```python
from build123d import *

# Parameters (mm, degrees)
SKETCH1_R           = 35
BOSS_EXTRUDE1_DEPTH = 170
SKETCH4_R           = 35
BOSS_EXTRUDE2_DEPTH = 85
SKETCH5_R           = 32.5
CUT_EXTRUDE2_DEPTH  = 85
SKETCH2_R           = 32.5
CUT_EXTRUDE3_DEPTH  = 194.261480901


with BuildPart() as part:
    # Sketch1 → Boss-Extrude1 (new body)
    with BuildSketch(Plane(origin=(0, 0, 0), x_dir=(0, 0, -1), z_dir=(1, 0, 0))):
        Circle(SKETCH1_R)
    extrude(amount=-BOSS_EXTRUDE1_DEPTH)

    # Sketch4 → Boss-Extrude2 (add)
    with BuildSketch(Plane.XY):
        with Locations((-85, 0)):
            Circle(SKETCH4_R)
    extrude(amount=-BOSS_EXTRUDE2_DEPTH)

    # Sketch5 → Cut-Extrude2 (cut)
    with BuildSketch(Plane(origin=(0, 0, -85), x_dir=(-1, 0, 0), z_dir=(0, 0, -1))):
        with Locations((85, 0)):
            Circle(SKETCH5_R)
    extrude(amount=-CUT_EXTRUDE2_DEPTH, mode=Mode.SUBTRACT)

    # Sketch2 → Cut-Extrude3 (cut, through all)
    with BuildSketch(Plane(origin=(0, 0, 0), x_dir=(0, 0, -1), z_dir=(1, 0, 0))):
        Circle(SKETCH2_R)
    extrude(amount=-CUT_EXTRUDE3_DEPTH, mode=Mode.SUBTRACT)


solid = part.part
```
Here's how the part is built. I have some questions about the finished solid (model axes, mm). A direction names the side the tool comes from. Round coordinates to 2 decimals unless told otherwise and drop trailing zeros. Write each loop counter-clockwise with the first axis right and the second up, starting at its lowest first coordinate (ties: lowest second). Pieces come first, ordered by that corner, then holes.
Q1. If we section it at A-A on y = 0: Write out the boundary of the cut face in (x, z), plus the area to 4 significant figures.
Q2. If we section it at D-D on y = -25: Write out the boundary of the cut face in (x, z), plus the area to 3 significant figures.
Q3. If we section it at C-C on z = -11.5: Write out the boundary of the cut face in (x, y), plus the area to 3 significant figures.
Q4. Will these pins go through, and if not, where does the flat tip stop? P1, Ø10, axis at x = -59, y = 14, coming from the +Z side; P2, Ø1, axis at x = -29.5, y = -25.5, coming from the -Z side; P3, Ø12, axis at y = 18.5, z = -12, coming from the -X side; P4, Ø5, axis at x = -60.5, z = -68.5, coming from the +Y side.
Q5. If we mould it in two halves opening along Y, with no side actions, what happens to faces 3 (the cylindrical face through (-83.81, 1.539, 34.966)), 4 (the flat face through (-61.8, -23.2, -85)), 5 (the cylindrical face through (-83.81, 1.43, 32.47))? For each: +Y half, -Y half, draft (parallel to the pull), parting line (faces both ways), or undercut.
Q6. Please list where these lines run through material, in increasing order: probe 1 along Y at (x, z) = (-85, -43); probe 2 along X at (y, z) = (0, -56.5); probe 3 along Y at (x, z) = (-141.5, -23).
Q7. Which directions (+Z, -Z, +X, -X, +Y, -Y) give clear straight access to the entire face, cutting with the end or side of a thin tool? Please do faces 1 (the flat face through (0, -23.2, -23.2)), 2 (the cylindrical face through (-80.769, 32.223, -52.539)).
Q8. If we section it at B-B on x = -113: Write out the boundary of the cut face in (y, z).
Answer below:
1. outline: (-170, -35) - (-120, -35) - (-120, -85) - (-117.5, -85) - (-117.5, -32.5) - (-170, -32.5) - close; (-170, 32.5) - (0, 32.5) - (0, 35) - (-170, 35) - close; (-52.5, -85) - (-50, -85) - (-50, -35) - (0, -35) - (0, -32.5) - (-52.5, -32.5) - close
1. area: 937.5 mm2
2. outline: (-170, -24.49) - (-109.49, -24.49) - (-109.49, -85) - (-105.77, -85) - (-105.77, -20.77) - (-170, -20.77) - close; (-170, 20.77) - (0, 20.77) - (0, 24.49) - (-170, 24.49) - close; (-64.23, -85) - (-60.51, -85) - (-60.51, -24.49) - (0, -24.49) - (0, -20.77) - (-64.23, -20.77) - close
2. area: 1,560 mm2
3. outline: (-170, -33.06) - (-96.5, -33.06) arc R35 ccw to (-73.5, -33.06) - (0, -33.06) - (0, -30.4) - (-73.5, -30.4) arc R32.5 cw to (-96.5, -30.4) - (-170, -30.4) - close; (-170, 30.4) - (-96.5, 30.4) arc R32.5 cw to (-73.5, 30.4) - (0, 30.4) - (0, 33.06) - (-73.5, 33.06) arc R35 ccw to (-96.5, 33.06) - (-170, 33.06) - close
3. area: 899 mm2
4. P1: stops at z = 33.82
4. P2: stops at z = -24.49
4. P3: passes through
4. P4: stops at y = 27.22
5. face 3: parting line
5. face 4: draft
5. face 5: undercut
6. probe 1: y = -35 to -32.5, 32.5 to 35
6. probe 2: x = -120 to -117.5, -52.5 to -50
6. probe 3: y = -26.38 to -22.96, 22.96 to 26.38
7. face 1: +Z, -Z, +X, +Y, -Y
7. face 2: -Z
8. outline: (-21, -85) - (-16.5, -85) - (-16.5, -28) arc R32.5 cw (long way) to (16.5, -28) - (16.5, -85) - (21, -85) - (21, -28) arc R35 ccw (long way) to (-21, -28) - close
